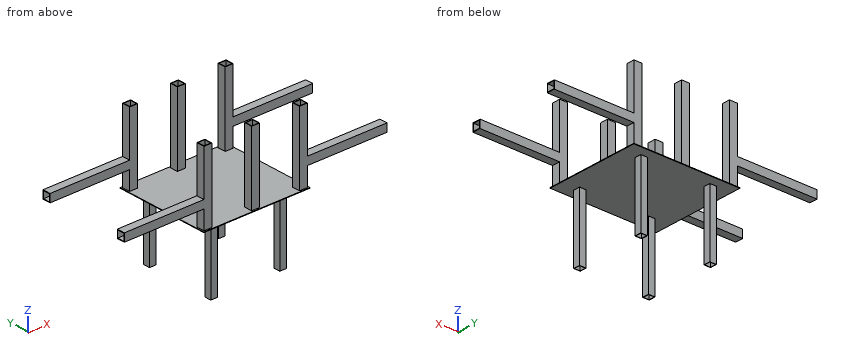
from build123d import *

# Parameters (mm, degrees)
SKETCH_1_W        = 30
SKETCH_1_H        = 30
SKETCH_1_W_2      = 26
SKETCH_1_H_2      = 26
EXTRUDE_1_DEPTH   = 270
EXTRUDE_1_2_DEPTH = 270
EXTRUDE_1_3_DEPTH = 270
EXTRUDE_1_4_DEPTH = 270
EXTRUDE_1_5_DEPTH = 270
EXTRUDE_1_6_DEPTH = 270
SKETCH_1_4_W      = 400
SKETCH_1_4_H      = 355
EXTRUDE_2_DEPTH   = 2
SKETCH_3_W        = 25
SKETCH_3_H        = 25
SKETCH_3_W_2      = 22
SKETCH_3_H_2      = 22
EXTRUDE_3_DEPTH   = 250
SKETCH_8_W        = 30
SKETCH_8_H        = 30
SKETCH_8_W_2      = 26
SKETCH_8_H_2      = 26
EXTRUDE_4_DEPTH   = 300


with BuildPart() as part:
    # Sketch 1 → Extrude 1 (new body)
    with BuildSketch(Plane.XY):
        with Locations((-139.865693992, 17.660065035)):
            Rectangle(SKETCH_1_W, SKETCH_1_H)
        with Locations((-139.865693992, 17.660065035)):
            Rectangle(SKETCH_1_W_2, SKETCH_1_H_2, mode=Mode.SUBTRACT)
    extrude(amount=EXTRUDE_1_DEPTH)



with BuildPart() as body_2:
    # Sketch 1 → Extrude 1 2 (new body)
    with BuildSketch(Plane.XY):
        with Locations((40.134306008, 17.660065035)):
            Rectangle(SKETCH_1_W, SKETCH_1_H)
        with Locations((40.134306008, 17.660065035)):
            Rectangle(SKETCH_1_W_2, SKETCH_1_H_2, mode=Mode.SUBTRACT)
    extrude(amount=EXTRUDE_1_2_DEPTH)


with BuildPart() as body_3:
    # Sketch 1 → Extrude 1 3 (new body)
    with BuildSketch(Plane.XY):
        with Locations((220.134306008, 17.660065035)):
            Rectangle(SKETCH_1_W, SKETCH_1_H)
        with Locations((220.134306008, 17.660065035)):
            Rectangle(SKETCH_1_W_2, SKETCH_1_H_2, mode=Mode.SUBTRACT)
    extrude(amount=EXTRUDE_1_3_DEPTH)


with BuildPart() as body_4:
    # Sketch 1 → Extrude 1 4 (new body)
    with BuildSketch(Plane.XY):
        with Locations((-139.865693992, -297.339934965)):
            Rectangle(SKETCH_1_W, SKETCH_1_H)
        with Locations((-139.865693992, -297.339934965)):
            Rectangle(SKETCH_1_W_2, SKETCH_1_H_2, mode=Mode.SUBTRACT)
    extrude(amount=EXTRUDE_1_4_DEPTH)


with BuildPart() as body_5:
    # Sketch 1 → Extrude 1 5 (new body)
    with BuildSketch(Plane.XY):
        with Locations((40.134306008, -297.339934965)):
            Rectangle(SKETCH_1_W, SKETCH_1_H)
        with Locations((40.134306008, -297.339934965)):
            Rectangle(SKETCH_1_W_2, SKETCH_1_H_2, mode=Mode.SUBTRACT)
    extrude(amount=EXTRUDE_1_5_DEPTH)


with BuildPart() as body_6:
    # Sketch 1 → Extrude 1 6 (new body)
    with BuildSketch(Plane.XY):
        with Locations((220.134306008, -297.339934965)):
            Rectangle(SKETCH_1_W, SKETCH_1_H)
        with Locations((220.134306008, -297.339934965)):
            Rectangle(SKETCH_1_W_2, SKETCH_1_H_2, mode=Mode.SUBTRACT)
    extrude(amount=EXTRUDE_1_6_DEPTH)


with BuildPart() as part_1:
    add(part.part)

    add(body_2.part)  # Extrude 2 merges body 2

    add(body_3.part)  # Extrude 2 merges body 3

    add(body_4.part)  # Extrude 2 merges body 4

    add(body_5.part)  # Extrude 2 merges body 5

    add(body_6.part)  # Extrude 2 merges body 6
    # Sketch 1_4 → Extrude 2 (add)
    with BuildSketch(Plane.XY):
        with Locations((40.134306008, -139.839934965)):
            Rectangle(SKETCH_1_4_W, SKETCH_1_4_H)
    extrude(amount=-EXTRUDE_2_DEPTH)

    # Sketch 3 → Extrude 3 (add)
    with BuildSketch(Plane(origin=(0, 0, -2), x_dir=(-1, 0, 0), z_dir=(0, 0, -1))):
        with Locations((-170.134306008, -9.839934965)):
            Rectangle(SKETCH_3_W, SKETCH_3_H)
        with Locations((-170.134306008, -9.839934965)):
            Rectangle(SKETCH_3_W_2, SKETCH_3_H_2, mode=Mode.SUBTRACT)
        with Locations((-170.134306008, -269.839934965)):
            Rectangle(SKETCH_3_W, SKETCH_3_H)
        with Locations((-170.134306008, -269.839934965)):
            Rectangle(SKETCH_3_W_2, SKETCH_3_H_2, mode=Mode.SUBTRACT)
        with Locations((89.865693992, -269.839934965)):
            Rectangle(SKETCH_3_W, SKETCH_3_H)
        with Locations((89.865693992, -269.839934965)):
            Rectangle(SKETCH_3_W_2, SKETCH_3_H_2, mode=Mode.SUBTRACT)
        with Locations((89.865693992, -9.839934965)):
            Rectangle(SKETCH_3_W, SKETCH_3_H)
        with Locations((89.865693992, -9.839934965)):
            Rectangle(SKETCH_3_W_2, SKETCH_3_H_2, mode=Mode.SUBTRACT)
    extrude(amount=EXTRUDE_3_DEPTH)

    # Sketch 8 → Extrude 4 (add)
    with BuildSketch(Plane.ZY.offset(154.865693992)):
        with Locations((85, -297.339934965)):
            Rectangle(SKETCH_8_W, SKETCH_8_H)
        with Locations((85, -297.339934965)):
            Rectangle(SKETCH_8_W_2, SKETCH_8_H_2, mode=Mode.SUBTRACT)
        with Locations((85, 17.660065035)):
            Rectangle(SKETCH_8_W, SKETCH_8_H)
        with Locations((85, 17.660065035)):
            Rectangle(SKETCH_8_W_2, SKETCH_8_H_2, mode=Mode.SUBTRACT)
    extrude_4 = extrude(amount=EXTRUDE_4_DEPTH)

    # Mirror 1: Extrude 4 across plane
    add(extrude_4.mirror(Plane.ZY.offset(-40.134306008)))


solid = part_1.part
Could you check a few things on this model? Use its own coordinates, in mm. Round coordinates to 2 decimals unless told otherwise and drop trailing zeros. Write each loop counter-clockwise with the first axis right and the second up, starting at its lowest first coordinate (ties: lowest second). Pieces come first, ordered by that corner, then holes. Notation, with made-up numbers: (25, 84.25) - (44, 84.25) arc R27 cw to (44, 119.25) - close; hole circle Ø8 at (62.5, 21.5). An arc over 180 degrees is marked (long way). Use a Markdown table: item, result.
Q1. I want a section at B-B (x = 436). List the corners of the cut face in (y, z) for me.
Output values:
| item | result |
|---|---|
| outline | (-312.34, 70) - (-282.34, 70) - (-282.34, 100) - (-312.34, 100) - close; (2.66, 70) - (32.66, 70) - (32.66, 100) - (2.66, 100) - close; hole (-310.34, 72) - (-284.34, 72) - (-284.34, 98) - (-310.34, 98) - close; hole (4.66, 72) - (30.66, 72) - (30.66, 98) - (4.66, 98) - close |
Q2. I want a section at D-D (y = -137.5). List the corners of the cut face in (x, z) for me, plus the area to 3 significant figures.
Output values:
| item | result |
|---|---|
| outline | (-159.87, -2) - (240.13, -2) - (240.13, 0) - (-159.87, 0) - close |
| area | 800 mm2 |
Q3. Please list where these lines run through material, in increasing order: L1, parallel to X at y = -4.5, z = -204; L2, parallel to X at y = 6, z = 203; L3, parallel to Y at x = 171, z = -48.
Output values:
| item | result |
|---|---|
| L1 | -102.37 to -100.87, -78.87 to -77.37, 157.63 to 159.13, 181.13 to 182.63 |
| L2 | -154.87 to -152.87, -126.87 to -124.87, 25.13 to 27.13, 53.13 to 55.13, 205.13 to 207.13, 233.13 to 235.13 |
| L3 | -282.34 to -280.84, -258.84 to -257.34, -22.34 to -20.84, 1.16 to 2.66 |
Q4. For pin 1 (12 mm diameter, centred on y = -17.5, z = -157.5, fed in from +X); pin 2 (11 mm diameter, centred on x = -84.5, z = -172, fed in from +Y); pin 3 (1.6 mm diameter, centred on y = -192, z = -0.5, fed in from -X), each with a flat end and sliding along its axis, tell me the tip position at first contact or that it passes through.
Output values:
| item | result |
|---|---|
| pin 1 | x = 182.63 |
| pin 2 | y = 2.66 |
| pin 3 | x = -159.87 |
Q5. I want a section at C-C (x = 40). List the corners of the cut face in (y, z) for me.
Output values:
| item | result |
|---|---|
| outline | (-317.34, -2) - (37.66, -2) - (37.66, 0) - (32.66, 0) - (32.66, 270) - (30.66, 270) - (30.66, 0) - (4.66, 0) - (4.66, 270) - (2.66, 270) - (2.66, 0) - (-282.34, 0) - (-282.34, 270) - (-284.34, 270) - (-284.34, 0) - (-310.34, 0) - (-310.34, 270) - (-312.34, 270) - (-312.34, 0) - (-317.34, 0) - close |
Q6. I want a section at A-A (z = -97.5). Count the separate pieces of the cut face and the enclosed holes in it, plus the area to 3 significant figures.
Output values:
| item | result |
|---|---|
| separate pieces | 4 |
| enclosed holes | 4 |
| area | 564 mm2 |
